from build123d import *

# Parameters (mm, degrees)
SKETCH_R        = 3.16
PAD_DEPTH       = 2.5
PAD001_DEPTH    = 20
SKETCH002_R     = 1.6
POCKET_DEPTH    = 4.061
FILLET_R        = 3
SKETCH003_W     = 9.48
SKETCH003_H     = 9.48
POCKET001_DEPTH = 1.56


with BuildPart() as part:
    # Sketch → Pad (new body)
    with BuildSketch(Plane.XY):
        with BuildLine():
            Line((-10, 10), (10, 10))
            Line((10, 10), (10, -10))
            Line((10, -10), (-10, -10))
            ThreePointArc((-10, 10), (-20, 0), (-10, -10))
        make_face()
        with Locations((-15, 0)):
            Circle(SKETCH_R, mode=Mode.SUBTRACT)
    extrude(amount=PAD_DEPTH)

    # Sketch001 (on Face3 of Pad) → Pad001 (join)
    with BuildSketch(Plane.XZ.offset(10)):
        Polygon((-4.74, 0), (4.74, 0), (2.94, -1.56), (-2.94, -1.56), align=None)
    extrude(amount=-PAD001_DEPTH)

    # Sketch002 (on Face11 of Pad001) → Pocket (cut, through all)
    with BuildSketch(Plane(origin=(0, 0, -1.56), x_dir=(1, 0, 0), z_dir=(0, 0, -1))):
        Circle(SKETCH002_R)
    extrude(amount=-POCKET_DEPTH, mode=Mode.SUBTRACT)

    # Fillet
    fillet_edges = [part.edges().sort_by_distance(p)[0] for p in [
        (10, -10, 1.25),
        (10, 10, 1.25),
    ]]
    fillet(fillet_edges, radius=FILLET_R)

    # Sketch003 (on Face13 of Fillet) → Pocket001 (cut)
    with BuildSketch(Plane(origin=(0, 0, -1.56), x_dir=(1, 0, 0), z_dir=(0, 0, -1))):
        Rectangle(SKETCH003_W, SKETCH003_H)
    extrude(amount=-POCKET001_DEPTH, mode=Mode.SUBTRACT)


solid = part.part
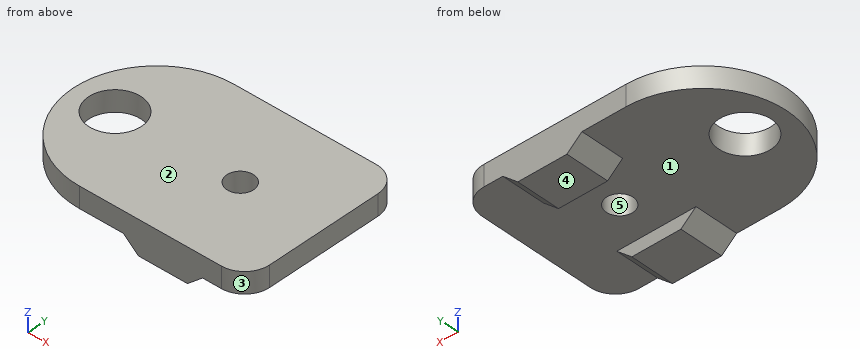
Input: part model. Units: mm. Frame: model coordinates. Face numbers are marked on the shaded views. A direction names the side the tool comes from. Give positions to 0.01 mm unless a question says otherwise; leave off trailing zeros. Write each loop counter-clockwise with the first axis right and the second up, starting at its lowest first coordinate (ties: lowest second). Pieces come first, ordered by that corner, then holes. Notation, with made-up numbers: M 73,-0.75 L 116,-0.75 A25 cw 116,24.25 Z; hole C 43,38.25 d11. An arc over 180 degrees is marked long. Use one line per item in the form item = value.
1. Mould query, pull axis X, two halves, no side actions, for the marked faces 3, 4 and 5. Classes: released by +X, released by -X, zero draft, split by the parting line, or undercut.
Outcome:
face_3 = released by +X
face_4 = zero draft
face_5 = undercut
2. Cut plane C-C on z = -0.55. Return loops of the section in (x, y), and give its area (3 significant figures).
Outcome:
outline = M -4.11,-10 L 4.11,-10 L 4.11,-4.74 L -4.11,-4.74 Z; M -4.11,4.74 L 4.11,4.74 L 4.11,10 L -4.11,10 Z
area = 86.4 mm²
3. Ray query, L1, parallel to Y at x = 0, z = 1.6; L2, parallel to X at y = 0.5, z = 1.4; L3, parallel to Y at x = -0.5, z = -1.3. Return the intervals inside material, ascending.
Outcome:
L1 = -10 to -1.6, 1.6 to 10
L2 = -19.99 to -18.12, -11.88 to -1.52, 1.52 to 10
L3 = -10 to -4.74, 4.74 to 10
4. Cut plane D-D on x = -15. Return loops of the section in (y, z), and give its area (3 significant figures).
Outcome:
outline = M -8.66,0 L -3.16,0 L -3.16,2.5 L -8.66,2.5 Z; M 3.16,0 L 8.66,0 L 8.66,2.5 L 3.16,2.5 Z
area = 27.5 mm²
5. Cut plane A-A on y = 0. Return loops of the section in (x, z), and give its area (3 significant figures).
Outcome:
outline = M -20,0 L -18.16,0 L -18.16,2.5 L -20,2.5 Z; M -11.84,0 L -1.6,0 L -1.6,2.5 L -11.84,2.5 Z; M 1.6,0 L 10,0 L 10,2.5 L 1.6,2.5 Z
area = 51.2 mm²
6. Reachability of the marked faces 1 and 2 from +Z, -Z, +X, -X, +Y, -Y: full face, straight path, thin tool, end or side. Return the list, or none.
Outcome:
face_1 = -Z
face_2 = +Z, +X, -X, +Y, -Y
7. Cut plane B-B on x = 0. Return loops of the section in (y, z).
Outcome:
outline = M -10,-1.56 L -4.74,-1.56 L -4.74,0 L -1.6,0 L -1.6,2.5 L -10,2.5 Z; M 1.6,0 L 4.74,0 L 4.74,-1.56 L 10,-1.56 L 10,2.5 L 1.6,2.5 Z
8. First-contact query: P1, Ø1, axis at x = 7, y = 5.5, coming from the -Z side; P2, Ø3, axis at x = 0, y = 0, coming from the +Z side. Flat tips, straight axial feed; report the tip coordinate or a pass-through.
Outcome:
P1 = 0
P2 = through
